from build123d import *

# Parameters (mm, degrees)
F0_R     = 60.325
F0_R_2   = 58.7375
F1_DEPTH = 3.175
F2_DEPTH = 9.525
F3_D     = 5.1054
F3_DEPTH = 76.2
F3_TIP   = 1.5338169022


# Not quite as in the source:
# - a feature names something its author has since deleted; it is built from what else it names


with BuildPart() as f1:
    # F0 (on Top) → F1 (new body)
    with BuildSketch(Plane.XY):
        Circle(F0_R)
        Circle(F0_R_2, mode=Mode.SUBTRACT)
        Circle(F0_R_2)
    extrude(amount=F1_DEPTH)

    # F0 (on Top) → F2 (join)
    with BuildSketch(Plane.XY):
        Circle(F0_R_2)
    extrude(amount=F2_DEPTH)

    # F3
    with Locations(Plane(origin=(0, 0, 0), x_dir=(1, 0, 0), z_dir=(0, 0, -1))):
        with Locations((38.1, -38.1), (-38.1, -38.1), (-38.1, 38.1), (38.1, 38.1)):
            Hole(F3_D / 2, depth=F3_DEPTH)
            with Locations((0, 0, -(F3_DEPTH + F3_TIP / 2))):  # 118° drill point
                Cone(0, F3_D / 2, F3_TIP, mode=Mode.SUBTRACT)


solid = f1.part
Input: part model. Units: mm. Frame: model coordinates. A direction names the side the tool comes from. Give positions to 0.01 mm unless a question says otherwise; leave off trailing zeros. Order: outer loops, then holes, each group sorted by start corner. A loop starts at its lowest first (then second) coordinate and runs counter-clockwise, first axis right, second up. Notation, with made-up numbers: (34.5, -24.75) - (72.5, -24.75) arc R18 ccw to (72.5, -6.75) - close; hole circle Ø7 at (-5.75, 6.25). An arc over 180 degrees is marked (long way). Write each question's results on one line, items separated by ' | '.
Item 1: Section B-B (y = 0). Return loops of the section in (x, z) (1 decimal).
A:
outline: (-60.3, 0) - (60.3, 0) - (60.3, 3.2) - (58.7, 3.2) - (58.7, 9.5) - (-58.7, 9.5) - (-58.7, 3.2) - (-60.3, 3.2) - close
Item 2: Material intervals for line 1 along Y through (x, z) = (-38.1, 3); line 2 along X through (y, z) = (-38.1, 7); line 3 along X through (y, z) = (-39.5, 8.25), sorted ascending.
A:
line 1: y = -46.77 to -40.65, -35.55 to 35.55, 40.65 to 46.77 | line 2: x = -44.7 to -40.65, -35.55 to 35.55, 40.65 to 44.7 | line 3: x = -43.47 to -40.23, -35.97 to 35.97, 40.23 to 43.47
Item 3: Contact query for flat-ended pins moving along their axis: pin 1 Ø12 at (x, y) = (-46.5, -19.5) entering from -Z; pin 2 Ø1.5 at (x, z) = (-1, 8.5) entering from +Y; pin 3 Ø1 at (y, z) = (-45.5, 2.5) entering from +X; pin 4 Ø1.5 at (y, z) = (-24, 1.5) entering from +X. Output: stop coordinate, or through.
A:
pin 1: stops at z = 0 | pin 2: stops at y = 58.74 | pin 3: stops at x = 40.18 | pin 4: stops at x = 55.66
Item 4: Section A-A (x = 37.5). Return loops of the section in (y, z) (3 decimals).
A:
outline: (-47.253, 0) - (-40.581, 0) - (-40.581, 9.525) - (-45.209, 9.525) - (-45.209, 3.175) - (-47.253, 3.175) - close; (-35.619, 0) - (35.619, 0) - (35.619, 9.525) - (-35.619, 9.525) - close; (40.581, 0) - (47.253, 0) - (47.253, 3.175) - (45.209, 3.175) - (45.209, 9.525) - (40.581, 9.525) - close
Item 5: Section D-D (y = 38.1). Return loops of the section in (x, z) (3 decimals), and give its area (3 significant figures).
A:
outline: (-46.771, 0) - (-40.653, 0) - (-40.653, 9.525) - (-44.704, 9.525) - (-44.704, 3.175) - (-46.771, 3.175) - close; (-35.547, 0) - (35.547, 0) - (35.547, 9.525) - (-35.547, 9.525) - close; (40.653, 0) - (46.771, 0) - (46.771, 3.175) - (44.704, 3.175) - (44.704, 9.525) - (40.653, 9.525) - close | area: 767 mm^2
Item 6: Draft query along Y for faces 3 (the cylindrical face through (-37.77, 35.57, 4.83)), 4 (the flat face through (-1, 1, 9.525)), 5 (the cylindrical face through (-60.267, 2.652, 1.565)). Return one class per face: released by +Y, released by -Y, zero draft, split by the parting line, or undercut.
A:
face 3: undercut | face 4: zero draft | face 5: split by the parting line
Item 7: Section C-C (z = 6.25). Return loops of the section in (x, y) (1 decimal), and give its area (3 significant figures).
A:
outline: circle Ø117.5 at (0, 0); hole circle Ø5.1 at (-38.1, -38.1); hole circle Ø5.1 at (-38.1, 38.1); hole circle Ø5.1 at (38.1, -38.1); hole circle Ø5.1 at (38.1, 38.1) | area: 10,800 mm^2
Item 8: Access query for faces 1 (the flat face through (-1, 1, 0)), 2 (the cylindrical face through (-46.612, -35.741, 6.306)). Directions: +Z, -Z, +X, -X, +Y, -Y. A direction counts if a zero-diameter tool reaches every point of the face in a straight line with its end or side. Return the directions, or none.
A:
face 1: -Z, +X, -X, +Y, -Y | face 2: +Z
